from build123d import *

# Parameters (mm, degrees)
F0_W     = 37.5
F0_H     = 15
F0_R     = 3.5
F0_R_2   = 2.6
F0_R_3   = 0.89
F1_DEPTH = 2.4


with BuildPart() as f1:
    # F0 (on Top) → F1 (new body)
    with BuildSketch(Plane.XY):
        with Locations((-50.939284, -7.5)):
            Rectangle(F0_W, F0_H)
        with Locations((-64.189284, -7.5)):
            Circle(F0_R, mode=Mode.SUBTRACT)
        with Locations((-49.689284, -7.5)):
            Circle(F0_R_2, mode=Mode.SUBTRACT)
        with Locations((-33.469284, -5)):
            Circle(F0_R_3, mode=Mode.SUBTRACT)
        with Locations((-13.439284, -7.5)):
            Rectangle(F0_W, F0_H)
        with Locations((-14.689284, -7.5)):
            Circle(F0_R_2, mode=Mode.SUBTRACT)
        with Locations((-30.909284, -5)):
            Circle(F0_R_3, mode=Mode.SUBTRACT)
        with Locations((-0.189284, -7.5)):
            Circle(F0_R, mode=Mode.SUBTRACT)
    extrude(amount=F1_DEPTH)


solid = f1.part
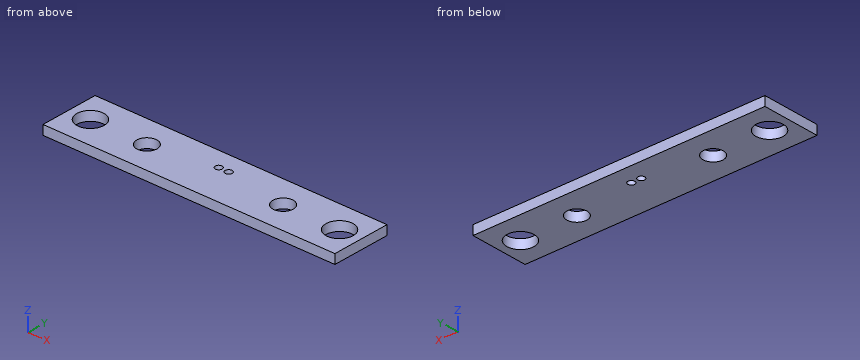
Geometry: final body of the model. Coordinates: model frame, mm. Give positions to 0.01 mm unless a question says otherwise; leave off trailing zeros. Loops run counter-clockwise (first coordinate to the right, second up) from the corner with the lowest first, then second, coordinate; pieces in that order, holes last. Notation, with made-up numbers: (50, 79) -> (88, 79) arc R23 ccw to (88, 105) -> close; hole circle Ø1 at (11.25, 49). An arc over 180 degrees is marked (long way). Put each result on its own line as item: value.
1. Cut plane C-C (x = -49.5). Return the cut outline in (y, z).
Taken from the geometry:
outline: (-15, 0) -> (-10.09, 0) -> (-10.09, 2.4) -> (-15, 2.4) -> close; (-4.91, 0) -> (0, 0) -> (0, 2.4) -> (-4.91, 2.4) -> close
2. Ray query, line 1 along X through (y, z) = (-7.75, 2.2); line 2 along X through (y, z) = (-6.25, 2); line 3 along Y through (x, z) = (-15.5, 1.2). Return the intervals inside material, ascending. Write a range as [from, to].
Taken from the geometry:
line 1: x = [-69.69, -67.68], [-60.7, -52.28], [-47.1, -17.28], [-12.1, -3.68], [3.3, 5.31]
line 2: x = [-69.69, -67.46], [-60.92, -51.97], [-47.41, -16.97], [-12.41, -3.46], [3.08, 5.31]
line 3: y = [-15, -9.97], [-5.03, 0]
3. Cut plane D-D (x = -16.5). Return the cut outline in (y, z), plus the area to 3 significant figures.
Taken from the geometry:
outline: (-15, 0) -> (-9.37, 0) -> (-9.37, 2.4) -> (-15, 2.4) -> close; (-5.63, 0) -> (0, 0) -> (0, 2.4) -> (-5.63, 2.4) -> close
area: 27.0 mm2
4. Cut plane A-A (y = -7.5). Return the cut outline in (x, z).
Taken from the geometry:
outline: (-69.69, 0) -> (-67.69, 0) -> (-67.69, 2.4) -> (-69.69, 2.4) -> close; (-60.69, 0) -> (-52.29, 0) -> (-52.29, 2.4) -> (-60.69, 2.4) -> close; (-47.09, 0) -> (-17.29, 0) -> (-17.29, 2.4) -> (-47.09, 2.4) -> close; (-12.09, 0) -> (-3.69, 0) -> (-3.69, 2.4) -> (-12.09, 2.4) -> close; (3.31, 0) -> (5.31, 0) -> (5.31, 2.4) -> (3.31, 2.4) -> close
5. Cut plane B-B (z = 0.55). Return the cut outline in (x, y).
Taken from the geometry:
outline: (-69.69, -15) -> (5.31, -15) -> (5.31, 0) -> (-69.69, 0) -> close; hole circle Ø7 at (-64.19, -7.5); hole circle Ø5.2 at (-49.69, -7.5); hole circle Ø1.78 at (-33.47, -5); hole circle Ø1.78 at (-30.91, -5); hole circle Ø5.2 at (-14.69, -7.5); hole circle Ø7 at (-0.19, -7.5)
